Read the model definition and answer for the solid it produces. Units are mm, in the model's axes. A direction names the side the tool comes from. Round coordinates to 2 decimals unless told otherwise and drop trailing zeros. Order: outer loops, then holes, each group sorted by start corner. A loop starts at its lowest first (then second) coordinate and runs counter-clockwise, first axis right, second up. Notation, with made-up numbers: (32, 45) -> (36, 45) arc R13 cw to (36, 62) -> close; hole circle Ø5 at (43, -3). An arc over 180 degrees is marked (long way). Use a Markdown table: item, result. Add a question column.
1. For faces 1 (the face through (-8, 1.647, 2)), 2 (the face through (1, -1, 1.25)), 3 (the face through (-11.544, 0, 2)), determine the directions among +Z, -Z, +X, -X, +Y, -Y from which every point of the face is accessible in a straight line to the end or side of a thin tool.
2. Section B-B, the plane z = 1.65 is taken. Give the vertices of the cut face in (x, y) (3 decimals).
3. Section D-D, the plane y = -0.75 is taken. Give the number of separate pieces and of enclosed holes in the cut face, then the cut area to 3 significant figures.
4. The mould has two halves that part along Y. Classify faces 4 (the face through (8, 1.75, 2)), 5 (the face through (-11.243, 2.94, 1.609)), 6 (the face through (-10.713, -2.419, 0.135)): +Y half, -Y half, draft (parallel to the pull), parting line (faces both ways), or undercut.
5. Section C-C, the plane x = -2.5 is taken. Give the vertices of the cut face in (y, z).
6. Given pin 1 (3 mm diameter, centred on x = 0, y = -0.32, fed in from -Z), flat-ended and moving along its own axis, determine where the tip first touches the part or whether it passes through.
7. Section A-A, the plane x = 8.25 is taken. Give the vertices of the cut face in (y, z), then the cut area to 3 significant figures.
8. Consider L1, parallel to X at y = 0, z = 0.55 (3 decimals); L2, parallel to X at y = -1.25, z = 1.8 (3 decimals); L3, parallel to Y at x = 0, z = 0.9. Determine where each line is inside the solid, lowest interval first. Write a range as [from, to].
```python
from build123d import *

# Parameters (mm, degrees)
PAD_DEPTH       = 3
CHAMFER_SIZE    = 0.5
SKETCH005_W     = 3.5
SKETCH005_H     = 3.5
POCKET_DEPTH    = 3.001
SKETCH003_R     = 1
POCKET004_DEPTH = 3.001
CHAMFER005_SIZE = 0.25
CHAMFER008_SIZE = 0.25
CHAMFER009_SIZE = 0.25
SKETCH010_R     = 1.75
POCKET005_DEPTH = 1.75
CHAMFER010_SIZE = 0.25
CHAMFER011_SIZE = 0.25


with BuildPart() as part:
    # Sketch → Pad (new body)
    with BuildSketch(Plane.XY):
        with BuildLine():
            Line((-9.543873, -3.274907), (9.456127, -3.274907))
            ThreePointArc((9.456127, -3.274907), (10.87034, -2.68912), (11.456127, -1.274907))
            Line((11.456127, -1.274907), (11.456127, 2.225093))
            ThreePointArc((11.456127, 2.225093), (11.163233, 2.9322), (10.456127, 3.225093))
            Line((-10.543873, 3.225093), (10.456127, 3.225093))
            ThreePointArc((-10.543873, 3.225093), (-11.25098, 2.9322), (-11.543873, 2.225093))
            Line((-11.543873, -1.274907), (-11.543873, 2.225093))
            ThreePointArc((-11.543873, -1.274907), (-10.958087, -2.68912), (-9.543873, -3.274907))
        make_face()
    extrude(amount=PAD_DEPTH)

    # Chamfer
    chamfer_edges = [part.edges().sort_by_distance(p)[0] for p in [
        (-0.043873, -3.274907, 0),
        (-10.958087, -2.68912, 0),
        (-10.543873, 3.225093, 1.5),
        (11.163233, 2.9322, 0),
        (11.456127, 0.475093, 0),
        (10.87034, -2.68912, 0),
    ]]
    chamfer(chamfer_edges, length=CHAMFER_SIZE)

    # Sketch005 (on DatumPlane) → Pocket (cut, through all)
    with BuildSketch(Plane.XY.offset(3)):
        with Locations((-8.14335, -0.103182)):
            Rectangle(SKETCH005_W, SKETCH005_H)
        with Locations((8.475, 0)):
            Rectangle(SKETCH005_W, SKETCH005_H)
    extrude(amount=-POCKET_DEPTH, mode=Mode.SUBTRACT)

    # Sketch003 (on DatumPlane) → Pocket004 (cut, through all)
    with BuildSketch(Plane.XY.offset(3)):
        with Locations((0, -0.324907)):
            Circle(SKETCH003_R)
    extrude(amount=-POCKET004_DEPTH, mode=Mode.SUBTRACT)

    # Chamfer005
    chamfer005_edges = [part.edges().sort_by_distance(p)[0] for p in [
        (11.456127, 0.475093, 3),
        (10.87034, -2.68912, 3),
        (-0.043873, -3.274907, 3),
        (-10.958087, -2.68912, 3),
        (-11.543873, 0.475093, 3),
        (-11.25098, 2.9322, 3),
        (-0.043873, 3.225093, 3),
        (11.163233, 2.9322, 3),
    ]]
    chamfer(chamfer005_edges, length=CHAMFER005_SIZE)

    # Chamfer008
    chamfer008_edges = [part.edges().sort_by_distance(p)[0] for p in [
        (8.475, -1.75, 0),
        (6.725, 0, 0),
        (8.475, 1.75, 0),
        (10.225, 0, 0),
        (-9.89335, -0.103182, 0),
        (-8.14335, 1.646818, 0),
        (-1, -0.324907, 0),
        (-6.39335, -0.103182, 0),
        (-8.14335, -1.853182, 0),
    ]]
    chamfer(chamfer008_edges, length=CHAMFER008_SIZE)

    # Chamfer009
    chamfer009_edges = [part.edges().sort_by_distance(p)[0] for p in [
        (6.725, 0, 3),
        (8.475, -1.75, 3),
        (10.225, 0, 3),
        (8.475, 1.75, 3),
        (-6.39335, -0.103182, 3),
        (-8.14335, -1.853182, 3),
        (-9.89335, -0.103182, 3),
        (-8.14335, 1.646818, 3),
    ]]
    chamfer(chamfer009_edges, length=CHAMFER009_SIZE)

    # Sketch010 (on Face10 of Chamfer009) → Pocket005 (cut)
    with BuildSketch(Plane.XY.offset(3)):
        with Locations((-0.025921, -0.324907)):
            Circle(SKETCH010_R)
    extrude(amount=-POCKET005_DEPTH, mode=Mode.SUBTRACT)

    # Chamfer010
    chamfer010_edges = [part.edges().sort_by_distance(p)[0] for p in [
        (-6.14335, -0.103182, 3),
    ]]
    chamfer(chamfer010_edges, length=CHAMFER010_SIZE)

    # Chamfer011
    chamfer011_edges = [part.edges().sort_by_distance(p)[0] for p in [
        (-1.775921, -0.324907, 3),
    ]]
    chamfer(chamfer011_edges, length=CHAMFER011_SIZE)


solid = part.part
```
Verdict:
| question | item | result |
|---|---|---|
| 1 | face 1 | +Z, -Z |
| 1 | face 2 | +Z |
| 1 | face 3 | +Z, -Z, -X, +Y, -Y |
| 2 | outline | (-11.544, -1.275) arc R2 ccw to (-9.544, -3.275) -> (9.456, -3.275) arc R2 ccw to (11.456, -1.275) -> (11.456, 2.225) arc R1 ccw to (10.456, 3.225) -> (-10.544, 3.225) arc R1 ccw to (-11.544, 2.225) -> close; hole (-9.893, -1.853) -> (-6.393, -1.853) -> (-6.393, 1.647) -> (-9.893, 1.647) -> close; hole circle Ø3.5 at (-0.026, -0.325); hole (6.725, -1.75) -> (10.225, -1.75) -> (10.225, 1.75) -> (6.725, 1.75) -> close |
| 3 | separate pieces | 4 |
| 3 | enclosed holes | 0 |
| 3 | area | 39.1 mm2 |
| 4 | face 4 | undercut |
| 4 | face 5 | +Y half |
| 4 | face 6 | -Y half |
| 5 | outline | (-3.27, 0.5) -> (-2.77, 0) -> (2.73, 0) -> (3.23, 0.5) -> (3.23, 2.75) -> (2.98, 3) -> (-3.02, 3) -> (-3.27, 2.75) -> close |
| 6 | pin 1 | stops at z = 0 |
| 7 | outline | (-3.27, 0.5) -> (-2.77, 0) -> (-2, 0) -> (-1.75, 0.25) -> (-1.75, 2.75) -> (-2, 3) -> (-3.02, 3) -> (-3.27, 2.75) -> close; (1.75, 0.25) -> (2, 0) -> (2.73, 0) -> (3.23, 0.5) -> (3.23, 2.75) -> (2.98, 3) -> (2, 3) -> (1.75, 2.75) -> close |
| 7 | area | 8.56 mm2 |
| 8 | L1 | x = [-11.544, -9.893], [-6.393, -0.946], [0.946, 6.725], [10.225, 11.456] |
| 8 | L2 | x = [-11.544, -9.893], [-6.393, -1.511], [1.46, 6.725], [10.225, 11.456] |
| 8 | L3 | y = [-3.27, -1.32], [0.68, 3.23] |
